from build123d import *

# Parameters (mm, degrees)
EXTRUDE_1_DEPTH          = 3.3
CUT_EXTRUDE_1_DEPTH      = 8.174566189
CUT_EXTRUDE_1_DEPTH_BACK = 8.174566189


with BuildPart() as part:
    # Эскиз1 → Бобышка-Вытянуть1 (new, symmetric)
    with BuildSketch(Plane(origin=(0, 0, 0), x_dir=(1, 0, 0), z_dir=(0, 1, 0))):
        with BuildLine():
            Line((-5.62, 0), (-3.95, 0))
            ThreePointArc((-3.95, 0), (-3.363101372, -0.243101372), (-3.12, -0.83))
            Line((-3.12, -0.83), (-3.12, -2.42))
            ThreePointArc((-3.12, -2.42), (-3.046776695, -2.596776695), (-2.87, -2.67))
            Line((-2.87, -2.67), (2.87, -2.67))
            ThreePointArc((2.87, -2.67), (3.046776695, -2.596776695), (3.12, -2.42))
            Line((3.12, -2.42), (3.12, -0.83))
            ThreePointArc((3.12, -0.83), (3.363101372, -0.243101372), (3.95, 0))
            Line((3.95, 0), (5.62, 0))
            Line((5.62, 0), (5.62, -0.33))
            Line((5.62, -0.33), (3.95, -0.33))
            ThreePointArc((3.95, -0.33), (3.596446609, -0.476446609), (3.45, -0.83))
            Line((3.45, -0.83), (3.45, -2.42))
            ThreePointArc((3.45, -2.42), (3.280121933, -2.830121933), (2.87, -3))
            Line((2.87, -3), (-2.87, -3))
            ThreePointArc((-2.87, -3), (-3.280121933, -2.830121933), (-3.45, -2.42))
            Line((-3.45, -2.42), (-3.45, -0.83))
            ThreePointArc((-3.45, -0.83), (-3.596446609, -0.476446609), (-3.95, -0.33))
            Line((-3.95, -0.33), (-5.62, -0.33))
            Line((-5.62, -0.33), (-5.62, 0))
        make_face()
    extrude(amount=EXTRUDE_1_DEPTH, both=True)

    # Эскиз2 → Вырез-Вытянуть1 (cut, two sides: drawn at the far end of the back side and taken through both)
    with BuildSketch(Plane(origin=(0, 0, 0), x_dir=(0, 0, -1), z_dir=(1, 0, 0)).offset(-CUT_EXTRUDE_1_DEPTH_BACK)):
        with BuildLine():
            Line((0, -1.5), (0, -2.4))
            Line((0, -2.4), (-1.8, -2.4))
            ThreePointArc((-1.8, -2.4), (-1.941421356, -2.341421356), (-2, -2.2))
            Line((-2, -2.2), (-2, -1.7))
            ThreePointArc((-2, -1.7), (-1.941421356, -1.558578644), (-1.8, -1.5))
            Line((-1.8, -1.5), (0, -1.5))
        make_face()
    extrude(amount=CUT_EXTRUDE_1_DEPTH + CUT_EXTRUDE_1_DEPTH_BACK, mode=Mode.SUBTRACT)


solid = part.part
Work out the finished part from the listing and answer in its coordinate system (mm). A direction names the side the tool comes from. Round coordinates to 2 decimals unless told otherwise and drop trailing zeros. Write each loop counter-clockwise with the first axis right and the second up, starting at its lowest first coordinate (ties: lowest second). Pieces come first, ordered by that corner, then holes.
1) A cutting plane is placed at B-B (z = 2.3). Give the vertices of the cut face in (x, y).
2) A cutting plane is placed at D-D (x = 3.25). Give the vertices of the cut face in (y, z).
3) Straight lines are drawn through the part: line 1 (X direction, y = -1.25, z = 0.8); line 2 (Z direction, x = 2.5, y = 2.75). For each, find the intervals that lie inside material, in ascending order.
4) A cutting plane is placed at A-A (z = 1). Give the vertices of the cut face in (x, y).
5) A tool of negligible diameter and unlimited length cuts with its end or side. For faces 1 (the flat face through (-5, -3, 0.33)), 2 (the flat face through (-5, 1, 0)), 3 (the flat face through (5, -3, 0.33)), 4 (the flat face through (0, 0, 2.67)), from which of +Z, -Z, +X, -X, +Y, -Y can it reach the whole face along a straight path? Write none if from no direction.
6) Given pin 1 Ø0.5 at (x, y) = (-5, 1) entering from +Z; pin 2 Ø1.5 at (x, y) = (-4.5, 2.5) entering from +Z; pin 3 Ø0.5 at (y, z) = (0, 2) entering from -X; pin 4 Ø0.9 at (x, z) = (-4.5, 0.5) entering from -Y, each flat-ended and moving along its own axis, determine where each tip first touches the part or whether it passes through.
7) A cutting plane is placed at C-C (y = -2). Give the vertices of the cut face in (x, z), plus the area to 3 significant figures.
Completed:
1. outline: (-3.45, -3.3) - (-3.12, -3.3) - (-3.12, 3.3) - (-3.45, 3.3) - close; (3.12, -3.3) - (3.45, -3.3) - (3.45, 3.3) - (3.12, 3.3) - close
2. outline: (-3.3, 0.38) - (-2.4, 0.38) - (-2.4, 1.8) arc R0.2 cw to (-2.2, 2) - (-1.7, 2) arc R0.2 cw to (-1.5, 1.8) - (-1.5, 0.38) - (3.3, 0.38) - (3.3, 2.86) - (-3.3, 2.86) - close
3. line 1: x = -3.45 to -3.12, 3.12 to 3.45
3. line 2: z = 2.67 to 3
4. outline: (-3.45, -3.3) - (-3.12, -3.3) - (-3.12, -2.4) - (-3.45, -2.4) - close; (-3.45, -1.5) - (-3.12, -1.5) - (-3.12, 3.3) - (-3.45, 3.3) - close; (3.12, -3.3) - (3.45, -3.3) - (3.45, -2.4) - (3.12, -2.4) - close; (3.12, -1.5) - (3.45, -1.5) - (3.45, 3.3) - (3.12, 3.3) - close
5. face 1: +Z, -X, +Y, -Y
5. face 2: -Z, +X, -X, +Y, -Y
5. face 3: +Z, +X, +Y, -Y
5. face 4: -Z, +Y, -Y
6. pin 1: stops at z = 0.33
6. pin 2: stops at z = 0.37
6. pin 3: stops at x = -3.45
6. pin 4: stops at y = -3.3
7. outline: (-3.45, 2) - (-3.12, 2) - (-3.12, 2.42) arc R0.25 cw to (-2.87, 2.67) - (2.87, 2.67) arc R0.25 cw to (3.12, 2.42) - (3.12, 2) - (3.45, 2) - (3.45, 2.42) arc R0.58 ccw to (2.87, 3) - (-2.87, 3) arc R0.58 ccw to (-3.45, 2.42) - close
7. area: 2.60 mm2
